Verification items for the finished model (mm, model axes). A direction names the side the tool comes from. Coordinates: 2 decimals unless noted, no trailing zeros. Write each loop counter-clockwise with the first axis right and the second up, starting at its lowest first coordinate (ties: lowest second). Pieces come first, ordered by that corner, then holes. Notation, with made-up numbers: (70, 37.25) -> (80, 37.25) arc R25 cw to (80, 68.25) -> close; hole circle Ø8 at (79.5, -10). An arc over 180 degrees is marked (long way). Answer in a Markdown table with one row per item.
Autodesk Inventor part; units mm, degrees
ref_plane "YZ Plane" through (0, 0, 0) normal (1, 0, 0) x (0, 1, 0)
ref_plane "XZ Plane" through (0, 0, 0) normal (0, 1, 0) x (-1, 0, 0)
ref_plane "XY Plane" through (0, 0, 0) normal (0, 0, 1) x (1, 0, 0)
sketch "Sketch1" plane through (0, 0, 0) normal (0, 0, 1) x (1, 0, 0)
  circle A0 centre (0, 0) radius 2
  dimension "d0" = 4
extrude "Extrusion1" add sketch "Sketch1" along normal blind 10
thread "Thread1"
sketch "Sketch2" plane through (0, 0, 0) normal (0, 1, 0) x (-1, 0, 0)
  line L0 (2, 0) -> (2, 10)
  line L1 (2, 0) -> (2, 0.5)
  line L2 (2, 0.5) -> (1.5, 0)
  line L3 (-2, 0) -> (2, 0)
  line L4 (2, 10) -> (-2, 10)
  line L5 (2, 10) -> (1.5, 10)
  line L6 (1.5, 10) -> (1.5, 9.5)
  line L7 (1.5, 9.5) -> (2, 9)
  line L8 (0, -2) -> (0, 12)
  point P0 (0, 0)
  dimension "d5" = 0.5
  dimension "d6" = 45
  dimension "d7" = 0.5
  dimension "d8" = 0.5
revolve "Revolution1" cut sketch "Sketch2" angle 360 about axis through (0, 0, -10) along (0, 0, 1) contours L3 L2 L0 | L7 L6 L4 L0
sketch "Sketch3" plane through (0, 0, 0) normal (0, 1, 0) x (-1, 0, 0)
  arc A0 (0, 10.8) -> (-1.1662, 10) centre (0, 9.55) ccw
  line L0 (1.5, 10) -> (-1.5, 10)
  line L1 (0, 10.8) -> (0, 10)
  line L2 (0, -2.1962) -> (0, 13.1769)
  point P0 (0, 0)
  dimension "d11" = 2.5
revolve "Revolution2" add sketch "Sketch3" angle 360 about axis through (0, 0, -10) along (0, 0, 1)
sketch "Sketch5" plane through (0, 0, 0) normal (0, 0, -1) x (-1, 0, 0)
  circle A0 centre (0, 0) radius 1
  line L0 (0.5774, -1) -> (-0.5774, -1)
  line L1 (-0.5774, -1) -> (-1.1547, 0)
  line L2 (0.5774, -1) -> (1.1547, 0)
  line L3 (0.5774, 1) -> (-0.5774, 1)
  line L4 (-0.5774, 1) -> (-1.1547, 0)
  line L5 (0.5774, 1) -> (1.1547, 0)
  dimension "d16" = 2
  dimension "d23" = 120
  dimension "d24" = 120
extrude "Extrusion2" cut sketch "Sketch5" against normal blind 2
sketch "Sketch7" plane through (0, 0, 0) normal (1, 0, 0) x (0, 1, 0)
  line L0 (0, 0) -> (0, 2)
  line L1 (-1, 0) -> (-1, 2)
  line L2 (0, 2) -> (-1, 2)
  line L3 (-1, 2) -> (0, 2.5774)
  line L4 (0, 2.5774) -> (0, 2)
  line L5 (0, -2.16) -> (0, 12.96)
  dimension "d28" = 60
revolve "Revolution3" cut sketch "Sketch7" angle 360 about axis through (0, 0, -10) along (0, 0, 1)
properties part number "wkret_z_kulka" material "Ogólne"
1. Access from +Z, -Z, +X, -X, +Y, -Y to the whole of each face (thin tool, end or side, straight path). Record for faces 3 (the face through (0.86, -0.51, 0.99)), 4 (the face through (0, 2, 5)).
Findings below:
| item | result |
|---|---|
| face 3 | -Z |
| face 4 | +Z, -Z |
2. Release check for a two-part mould opening along X. For faces 1 (the face through (0.86, 0.51, 0.99)), 2 (the face through (1.5, 0.07, 9.75)) record: released by +X, released by -X, zero draft, split by the parting line, or undercut.
Findings below:
| item | result |
|---|---|
| face 1 | undercut |
| face 2 | split by the parting line |
3. Sectioned sample at A-A, the plane z = 1.75. Record the cut outline in (x, y), and give its area (3 significant figures).
Findings below:
| item | result |
|---|---|
| outline | circle Ø4 at (0, 0); hole (-1.15, 0) -> (-0.58, -1) -> (0.58, -1) -> (1.15, 0) -> (0.58, 1) -> (-0.58, 1) -> close |
| area | 9.10 mm² |
4. Material ranges on probe 1 along Y at (x, z) = (-0.1, 0.75); probe 2 along Z at (x, y) = (-0.05, -1.25); probe 3 along X at (y, z) = (0.85, 1.75), recorded low to high. Write a range as from..to.
Findings below:
| item | result |
|---|---|
| probe 1 | y = -2..-1, 1..2 |
| probe 2 | z = 0..10 |
| probe 3 | x = -1.81..-0.66, 0.66..1.81 |
5. Sectioned sample at B-B, the plane z = 5. Record the cut outline in (x, y).
Findings below:
| item | result |
|---|---|
| outline | circle Ø4 at (0, 0) |
